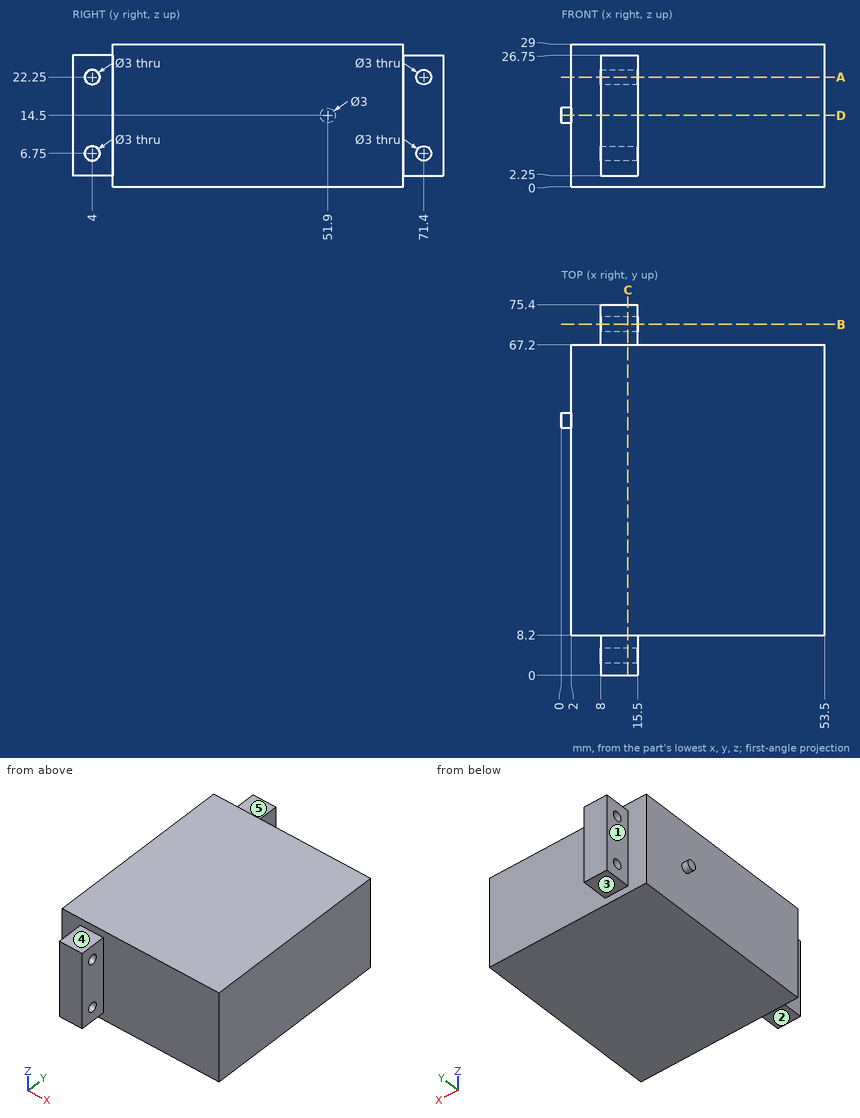
Geometry check sheet. Reference: drawing and pictorial views, mm from the part's lowest x, y, z. A direction names the side the tool comes from. Give positions to 0.01 mm unless a question says otherwise; leave off trailing zeros. Order: outer loops, then holes, each group sorted by start corner. A loop starts at its lowest first (then second) coordinate and runs counter-clockwise, first axis right, second up. Notation, with made-up numbers: M -32,8.25 L 15,8.25 A31 ccw 15,43.25 Z; hole C -22,-30.5 d4. An arc over 180 degrees is marked long. Answer as CSV lines item,"result". Start each with the question number.
Item 1: Cross-section at D-D on z = 14.5. Enter the section's corners in (x, y).
Item 2: Tool access check on the marked faces 1, 2, 3, 4 and 5. Record the directions out of +Z, -Z, +X, -X, +Y, -Y that give a thin tool (end or side, any length) a straight path to the whole face; none if there is none.
Item 3: Cross-section at B-B on y = 71.4. Enter the section's corners in (x, z), plus the area to 3 significant figures.
Item 4: Thickness scan on line 1 (Z direction, x = 10, y = 4); line 2 (Y direction, x = 10, z = 22.25); line 3 (Y direction, x = 27, z = 8.5). Record the ranges inside material, lowest first. Write a range as [from, to].
Item 5: Cross-section at C-C on x = 13.5. Enter the section's corners in (y, z).
Item 6: Gauge pin test, flat ends, axial feed: P1, Ø2, axis at x = 12.5, y = 5.5, coming from the +Z side; P2, Ø2.5, axis at y = 2, z = 19, coming from the +X side; P3, Ø10, axis at x = 15, y = 10, coming from the -Z side; P4, Ø1.8, axis at y = 71.4, z = 22.25, coming from the -X side. Record the tip position at first contact, or that the pin passes through.
Item 7: Cross-section at A-A on z = 22.25. Enter the section's corners in (x, y), plus the area to 3 significant figures.
Established:
1,outline,"M 0,50.4 L 2,50.4 L 2,8.2 L 8,8.2 L 8,0 L 15.5,0 L 15.5,8.2 L 53.5,8.2 L 53.5,67.2 L 15.5,67.2 L 15.5,75.4 L 8,75.4 L 8,67.2 L 2,67.2 L 2,53.4 L 0,53.4 Z"
2,face 1,"+Z, -Z, -X, +Y"
2,face 2,"-Z, +X, -X, -Y"
2,face 3,"-Z, +X, -X, +Y"
2,face 4,"+Z, +X, -X, -Y"
2,face 5,"+Z, +X, -X, +Y"
3,outline,"M 8,2.25 L 15.5,2.25 L 15.5,5.25 L 8,5.25 Z; M 8,8.25 L 15.5,8.25 L 15.5,20.75 L 8,20.75 Z; M 8,23.75 L 15.5,23.75 L 15.5,26.75 L 8,26.75 Z"
3,area,"139 mm^2"
4,line 1,"z = [2.25, 5.25], [8.25, 20.75], [23.75, 26.75]"
4,line 2,"y = [0, 2.5], [5.5, 69.9], [72.9, 75.4]"
4,line 3,"y = [8.2, 67.2]"
5,outline,"M 0,2.25 L 8.2,2.25 L 8.2,0 L 67.2,0 L 67.2,2.25 L 75.4,2.25 L 75.4,26.75 L 67.2,26.75 L 67.2,29 L 8.2,29 L 8.2,26.75 L 0,26.75 Z; hole C 4,6.75 d3; hole C 4,22.25 d3; hole C 71.4,6.75 d3; hole C 71.4,22.25 d3"
6,P1,"stops at z = 26.75"
6,P2,"stops at x = 15.5"
6,P3,"stops at z = 0"
6,P4,"passes through"
7,outline,"M 2,8.2 L 8,8.2 L 8,5.5 L 15.5,5.5 L 15.5,8.2 L 53.5,8.2 L 53.5,67.2 L 15.5,67.2 L 15.5,69.9 L 8,69.9 L 8,67.2 L 2,67.2 Z; M 8,0 L 15.5,0 L 15.5,2.5 L 8,2.5 Z; M 8,72.9 L 15.5,72.9 L 15.5,75.4 L 8,75.4 Z"
7,area,"3,120 mm^2"
